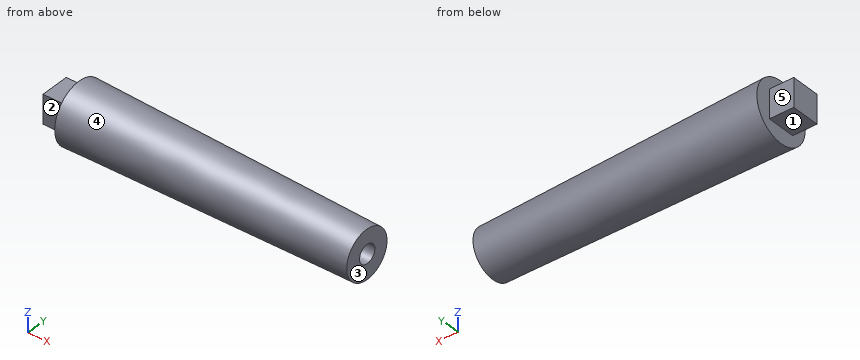
```python
from build123d import *

# Parameters (mm, degrees)
SKETCH4_R           = 4.826
CUT_EXTRUDE1_DEPTH  = 12.7
SKETCH6_R           = 15.875
CUT_EXTRUDE2_DEPTH  = 12.7
SKETCH8_W           = 14.986
SKETCH8_H           = 14.986
BOSS_EXTRUDE1_DEPTH = 12.7


with BuildPart() as part:
    # Sketch3 → Revolve5 (revolve)
    with BuildSketch(Plane.XY, mode=Mode.PRIVATE) as revolve5_sk:
        Polygon((0, 0), (165.1, 0), (165.1, 12.7), (0, 15.875), align=None)
    revolve(revolve5_sk.sketch.rotate(Axis((165.1, 12.7, 0), (-0.9998151400298467, 0.01922721423134321, 0)), 180), axis=Axis((165.1, 12.7, 0), (-0.9998151400298467, 0.01922721423134321, 0)))

    # Sketch4 → Cut-Extrude1 (cut, symmetric)
    with BuildSketch(Plane(origin=(165.1, 0, 0), x_dir=(0, 0, -1), z_dir=(1, 0, 0))):
        with Locations((0, 13.089439927)):
            Circle(SKETCH4_R)
    extrude(amount=CUT_EXTRUDE1_DEPTH, both=True, mode=Mode.SUBTRACT)

    # Sketch6 → Cut-Extrude2 (cut)
    with BuildSketch(Plane(origin=(0, 0, 0), x_dir=(0, 0, -1), z_dir=(1, 0, 0))):
        with Locations((0, 15.875)):
            Circle(SKETCH6_R)
    extrude(amount=CUT_EXTRUDE2_DEPTH, mode=Mode.SUBTRACT)

    # Sketch8 → Boss-Extrude1 (add)
    with BuildSketch(Plane.ZY.offset(-12.7)):
        with Locations((0, 15.636551979)):
            Rectangle(SKETCH8_W, SKETCH8_H)
    extrude(amount=BOSS_EXTRUDE1_DEPTH)


solid = part.part
```
Work out the finished part from the listing and answer in its coordinate system (mm). Face numbers are marked on the shaded views. A direction names the side the tool comes from. Give positions to 0.01 mm unless a question says otherwise; leave off trailing zeros. One line per item, written item: value. Start each with the question number.
1. Each of these flat-tipped pins is pushed along its axis until it touches: P1, Ø2, axis at x = 108.5, z = 8.5, coming from the -Y side; P2, Ø10, axis at x = 4.5, y = 13, coming from the +Z side; P3, Ø10, axis at x = 6, y = 13.5, coming from the -Z side. Where does it stop, or does it pass through?
2. Which of the six approach directions +Z, -Z, +X, -X, +Y, -Y give full straight-line access (tool end or side, diameter ignored) to the marked faces 4 and 5?
3. Find the intervals of material crossed by probe 1 along X at (y, z) = (16.5, -5.5); probe 2 along X at (y, z) = (17, 1.5); probe 3 along Z at (x, y) = (131, 20.5), in increasing order.
4. Determine the mould class of the marked faces 1, 2 and 3 for opening direction Z: released by +Z, released by -Z, zero draft, split by the parting line, or undercut.
Reported:
1. P1: stops at y = 2.22
1. P2: stops at z = 7.49
1. P3: stops at z = -7.49
2. face 4: +X
2. face 5: +Z, -Z, -X, +Y
3. probe 1: x = 0 to 165.3
3. probe 2: x = 0 to 152.4
3. probe 3: z = -11.29 to 11.29
4. face 1: released by -Z
4. face 2: zero draft
4. face 3: undercut
